Design review of the part built by this model. Coordinates are the model's own, in mm. A direction names the side the tool comes from. Round coordinates to 2 decimals unless told otherwise and drop trailing zeros. Order: outer loops, then holes, each group sorted by start corner. A loop starts at its lowest first (then second) coordinate and runs counter-clockwise, first axis right, second up. Notation, with made-up numbers: M -17,3 L -9,3 A25 ccw -9,40 Z; hole C 36.25,27.25 d8. An arc over 180 degrees is marked long. Use a Markdown table: item, result. Add a question column.
(1) Take a section at C-C (z = 5.5). Write out the cut boundary in (x, y).
(2) For pin 1 (2 mm diameter, centred on y = -3.5, z = -9, fed in from -X); pin 2 (16 mm diameter, centred on y = -61.5, z = 3, fed in from +X); pin 3 (1.5 mm diameter, centred on x = 2.5, z = 4.5, fed in from +Y), all flat-tipped, find the tip position at first contact; note any pin that passes through.
(3) Take a section at A-A (y = -54). Write out the cut boundary in (x, z).
(4) The part is to be moulded in two halves that separate along Z. For faces 1 (the face through (0, 16, 0)), 2 (the face through (-2, 0, 3)), 3 (the face through (-3, -39, 0)), 4 (the face through (0, -41, -16)), say which applies: released by +Z, released by -Z, zero draft, split by the parting line, or undercut.
(5) Take a section at B-B (x = 2). Count the separate pieces of the cut face and the enclosed holes in it, then the cut area to 3 significant figures.
(6) Machinability: for faces 5 (the face through (-2.51, -10.74, 2.38)), 6 (the face through (0, -39, 16)), 7 (the face through (3.49, -10.74, 2.38)), 8 (the face through (0.042, -61.064, 4.941)), 9 (the face through (0, -96, 0)), which of the approach directions +Z, -Z, +X, -X, +Y, -Y give a long, thin tool a straight path to every point of the face, cutting with its end or side? Answer none if there is none.
(7) To check wall thickness, follow probe 1 along Y at (x, z) = (0.65, 0); probe 2 along Y at (x, z) = (-2.5, 0); probe 3 along Y at (x, z) = (1.5, 7). State the ranges of each line that lie inside material, in increasing order. Write a range as from..to.
(8) Take a section at D-D (y = -14). Write out the cut boundary in (x, z).
```python
from build123d import *

# Parameters (mm, degrees)
BOSS_EXTRUDE1_DEPTH      = 3
BOSS_EXTRUDE1_DEPTH_BACK = 3
SKETCH1_R                = 11
BOSS_EXTRUDE2_DEPTH      = 4
BOSS_EXTRUDE2_DEPTH_BACK = 2
SKETCH1_2_R              = 11
CUT_EXTRUDE1_DEPTH       = 6
SKETCH3_R                = 2.5
SKETCH3_R_2              = 0.5
CUT_EXTRUDE2_DEPTH       = 6


with BuildPart() as part:
    # Sketch1 → Boss-Extrude1 (new, two sides: drawn at the far end of the back side and taken through both)
    with BuildSketch(Plane(origin=(0, 0, 0), x_dir=(0, 0, -1), z_dir=(1, 0, 0)).offset(-BOSS_EXTRUDE1_DEPTH_BACK)):
        with BuildLine():
            Line((-16, 0), (-16, -80))
            ThreePointArc((-16, -80), (0, -96), (16, -80))
            Line((16, -80), (16, 0))
            ThreePointArc((16, 0), (0, 16), (-16, 0))
        make_face()
        Circle(SKETCH1_R, mode=Mode.SUBTRACT)
        with Locations((0, -80)):
            Circle(SKETCH1_R, mode=Mode.SUBTRACT)
    extrude(amount=BOSS_EXTRUDE1_DEPTH + BOSS_EXTRUDE1_DEPTH_BACK)

    # Sketch1<2> → Boss-Extrude2 (add, two sides: drawn at the far end of the back side and taken through both)
    with BuildSketch(Plane(origin=(0, 0, 0), x_dir=(0, 0, -1), z_dir=(1, 0, 0)).offset(-BOSS_EXTRUDE2_DEPTH_BACK)):
        Circle(SKETCH1_2_R)
    extrude(amount=BOSS_EXTRUDE2_DEPTH + BOSS_EXTRUDE2_DEPTH_BACK)

    # Sketch2 → Cut-Extrude1 (cut)
    with BuildSketch(Plane(origin=(3, 0, 0), x_dir=(0, 0, -1), z_dir=(1, 0, 0))):
        with BuildLine():
            Line((-2.317597737, -26.071446828), (-2.317597737, -58.382201359))
            ThreePointArc((-2.317597737, -58.382201359), (-5, -61.064603622), (-7.682402263, -58.382201359))
            Line((-7.682402263, -58.382201359), (-7.682402263, -26.071446828))
            ThreePointArc((-7.682402263, -26.071446828), (-5, -23.389044565), (-2.317597737, -26.071446828))
        make_face()
        with BuildLine():
            Line((2.317597737, -26.071446828), (2.317597737, -58.382201359))
            ThreePointArc((2.317597737, -58.382201359), (5, -61.064603622), (7.682402263, -58.382201359))
            Line((7.682402263, -58.382201359), (7.682402263, -26.071446828))
            ThreePointArc((7.682402263, -26.071446828), (5, -23.389044565), (2.317597737, -26.071446828))
        make_face()
    extrude(amount=-CUT_EXTRUDE1_DEPTH, mode=Mode.SUBTRACT)

    # Sketch3 → Cut-Extrude2 (cut)
    with BuildSketch(Plane.ZY.offset(2)):
        Circle(SKETCH3_R)
        with Locations((0, 7)):
            Circle(SKETCH3_R_2)
        with Locations((-7, 0)):
            Circle(SKETCH3_R_2)
        with Locations((7, 0)):
            Circle(SKETCH3_R_2)
        with Locations((0, -7)):
            Circle(SKETCH3_R_2)
    extrude(amount=-CUT_EXTRUDE2_DEPTH, mode=Mode.SUBTRACT)


solid = part.part
```
Verdict:
| question | item | result |
|---|---|---|
| 1 | outline | M -3,-95.02 L 3,-95.02 L 3,-89.53 L -3,-89.53 Z; M -3,-70.47 L 3,-70.47 L 3,-61.02 L -3,-61.02 Z; M -3,-23.44 L 3,-23.44 L 3,-9.53 L 4,-9.53 L 4,9.53 L 3,9.53 L 3,15.02 L -3,15.02 L -3,9.53 L -2,9.53 L -2,-9.53 L -3,-9.53 Z |
| 2 | pin 1 | stops at x = -2 |
| 2 | pin 2 | stops at x = 3 |
| 2 | pin 3 | stops at y = 15.55 |
| 3 | outline | M -3,-16 L 3,-16 L 3,-7.68 L -3,-7.68 Z; M -3,-2.32 L 3,-2.32 L 3,2.32 L -3,2.32 Z; M -3,7.68 L 3,7.68 L 3,16 L -3,16 Z |
| 4 | face 1 | split by the parting line |
| 4 | face 2 | undercut |
| 4 | face 3 | zero draft |
| 4 | face 4 | released by -Z |
| 5 | separate pieces | 1 |
| 5 | enclosed holes | 8 |
| 5 | area | 2,570 mm^2 |
| 6 | face 5 | -X |
| 6 | face 6 | +Z, +X, -X, +Y, -Y |
| 6 | face 7 | +X |
| 6 | face 8 | +X, -X |
| 6 | face 9 | +X, -X, -Y |
| 7 | probe 1 | y = -96..-91, -69..-7.5, -6.5..-2.5, 2.5..6.5, 7.5..16 |
| 7 | probe 2 | y = -96..-91, -69..-11, 11..16 |
| 7 | probe 3 | y = -94.39..-88.49, -71.51..-60.17, -24.28..-0.5, 0.5..14.39 |
| 8 | outline | M -3,-16 L 3,-16 L 3,16 L -3,16 Z |
